from build123d import *

# Parameters (mm, degrees)
CROQUIS1_W              = 59.8
CROQUIS1_H              = 59.8
CROQUIS1_W_2            = 20.2
CROQUIS1_H_2            = 28.5
SALIENTE_EXTRUIR1_DEPTH = 10
CROQUIS1_3_W            = 20.2
CROQUIS1_3_H            = 28.5
CORTAR_EXTRUIR1_DEPTH   = 10
CROQUIS1_4_W            = 80
CROQUIS1_4_H            = 80
CROQUIS1_4_W_2          = 59.8
CROQUIS1_4_H_2          = 59.8
SALIENTE_EXTRUIR2_DEPTH = 5
CHAFL_N2_START          = -40
CHAFL_N2_DEPTH          = 80
CHAFL_N2_START_2        = -41
CHAFL_N2_2_DEPTH        = 82


with BuildPart() as part:
    # Croquis1 → Saliente-Extruir1 (new body)
    # profile 1 of 2: a face of its own
    with BuildSketch(Plane.XY):
        Rectangle(CROQUIS1_W, CROQUIS1_H)
        Rectangle(CROQUIS1_W_2, CROQUIS1_H_2, mode=Mode.SUBTRACT)
    # profile 2 of 2: a face of its own
    with BuildSketch(Plane.XY):
        Rectangle(CROQUIS1_W_2, CROQUIS1_H_2)
    extrude(amount=-SALIENTE_EXTRUIR1_DEPTH)

    # Croquis1<3> → Cortar-Extruir1 (cut)
    with BuildSketch(Plane.XY):
        Rectangle(CROQUIS1_3_W, CROQUIS1_3_H)
    extrude(amount=-CORTAR_EXTRUIR1_DEPTH, mode=Mode.SUBTRACT)

    # Croquis1<4> → Saliente-Extruir2 (add)
    with BuildSketch(Plane.XY):
        Rectangle(CROQUIS1_4_W, CROQUIS1_4_H)
        Rectangle(CROQUIS1_4_W_2, CROQUIS1_4_H_2, mode=Mode.SUBTRACT)
    extrude(amount=-SALIENTE_EXTRUIR2_DEPTH)

    # Chaflán2: read off the stored shape, not the designer's step
    # Chaflán2 outline → Chaflán2 (cut)
    with BuildSketch(Plane(origin=(0, 0, 0), x_dir=(1, 0, 0), z_dir=(0, 1, 0)).offset(CHAFL_N2_START)):
        Polygon((-40, 5), (-40, 0), (-37, 5), align=None)
        Polygon((40, 5), (37, 5), (40, 0), align=None)
    extrude(amount=CHAFL_N2_DEPTH, mode=Mode.SUBTRACT)

    # Chafl_n2 2 outline → Chafl_n2 2 (cut)
    with BuildSketch(Plane.YZ.offset(CHAFL_N2_START_2)):
        Polygon((40, -5), (40, 0), (37, -5), align=None)
        Polygon((-40, -5), (-37, -5), (-40, 0), align=None)
    extrude(amount=CHAFL_N2_2_DEPTH, mode=Mode.SUBTRACT)


solid = part.part
CAD build for the part. Positions are in the model's coordinates, mm. A direction names the side the tool comes from. Round coordinates to 2 decimals unless told otherwise and drop trailing zeros. Loops run counter-clockwise (first coordinate to the right, second up) from the corner with the lowest first, then second, coordinate; pieces in that order, holes last. Notation, with made-up numbers: (-5.75, -35) - (0.25, -35) arc R25 ccw to (0.25, -4) - close; hole circle Ø6 at (-0.5, 87). An arc over 180 degrees is marked (long way). Put each result on its own line as item: value.
1. 3-axis set-ups, long thin cutter, end or side, ignore diameter. For faces 4 (the flat face through (0, -29.9, -7)), 5 (the flat face through (-29.9, 0, -7)), 6 (the flat face through (0, -14.25, -5)): which of +Z, -Z, +X, -X, +Y, -Y reach the whole face in a straight line?
Geometry check:
face 4: -Z, +X, -X, -Y
face 5: -Z, -X, +Y, -Y
face 6: +Z, -Z
2. Slice it at A-A on y = -11.5. List the corners of the cut face in (x, z), and give its area (3 significant figures).
Geometry check:
outline: (-40, 0) - (-37, -5) - (-29.9, -5) - (-29.9, -10) - (-10.1, -10) - (-10.1, 0) - close; (10.1, -10) - (29.9, -10) - (29.9, -5) - (37, -5) - (40, 0) - (10.1, 0) - close
area: 482 mm²
3. Two-plate mould, pull along X, no slides. Class faces 1 (the flat face through (-38.5, -0.6, -2.5)), 2 (the flat face through (10.1, 0, -5)), 3 (the flat face through (0, 29.9, -7)): released by +X, released by -X, zero draft, split by the parting line, or undercut.
Geometry check:
face 1: released by -X
face 2: undercut
face 3: zero draft
4. Pin check, flat tips, straight feed: P1, Ø6, axis at y = -14.5, z = -7.5, coming from the -X side; P2, Ø2.5, axis at x = -6.5, z = -7.5, coming from the -Y side; P3, Ø5.5, axis at y = 3, z = -7, coming from the +X side. Stop position of each tip, or through.
Geometry check:
P1: x = -37.3
P2: y = -29.9
P3: x = 37.45
5. Slice it at D-D on x = 27. List the corners of the cut face in (y, z), and give its area (3 significant figures).
Geometry check:
outline: (-40, 0) - (-37, -5) - (-29.9, -5) - (-29.9, -10) - (29.9, -10) - (29.9, -5) - (37, -5) - (40, 0) - close
area: 684 mm²
6. Wall check: line 1 (Y direction, x = -6, z = -5.5); line 2 (Z direction, x = 35, y = -25); line 3 (X direction, y = -18, z = -6.5). Give the ranges that are in metal, low to high.
Geometry check:
line 1: -29.9 to -14.25, 14.25 to 29.9
line 2: -5 to 0
line 3: -29.9 to 29.9
7. Slice it at B-B on z = -3.5. List the corners of the cut face in (x, y).
Geometry check:
outline: (-37.9, -37.9) - (37.9, -37.9) - (37.9, 37.9) - (-37.9, 37.9) - close; hole (-10.1, -14.25) - (10.1, -14.25) - (10.1, 14.25) - (-10.1, 14.25) - close
8. Slice it at C-C on x = 7. List the corners of the cut face in (y, z).
Geometry check:
outline: (-40, 0) - (-37, -5) - (-29.9, -5) - (-29.9, -10) - (-14.25, -10) - (-14.25, 0) - close; (14.25, -10) - (29.9, -10) - (29.9, -5) - (37, -5) - (40, 0) - (14.25, 0) - close
